from build123d import *

# Parameters (mm, degrees)
F1_W     = 100
F1_H     = 10
F2_DEPTH = 10
F3_R     = 2
F5_COUNT = 4
F6_W     = 15
F6_H     = 15
F6_W_2   = 10
F6_H_2   = 10
F7_DEPTH = 10
F8_DEPTH = 25.4


with BuildPart() as f2:
    # F1 (on Top) → F2 (new body)
    with BuildSketch(Plane.XY):
        Rectangle(F1_W, F1_H)
    extrude(amount=F2_DEPTH)

    # F3
    f3_edges = [f2.edges().sort_by_distance(p)[0] for p in [
        (50, -5, 5),
        (50, 5, 5),
        (50, 0, 0),
        (50, 0, 10),
        (-50, 5, 5),
        (-50, -5, 5),
        (-50, 0, 0),
        (-50, 0, 10),
    ]]
    fillet(f3_edges, radius=F3_R)

    # F5: F2 ×4 about axis
    f5_axis = Axis((0, 0, 17.9461631924), (0, 0, 1))


with BuildPart() as f2_1:
    add(f2.part)
    for i in range(1, F5_COUNT):
        add(f2.part.rotate(f5_axis, i * 360 / F5_COUNT))

    # F6 (on Top) → F7 (join)
    with BuildSketch(Plane.XY):
        Rectangle(F6_W, F6_H)
        Rectangle(F6_W_2, F6_H_2, mode=Mode.SUBTRACT)
    extrude(amount=F7_DEPTH)

    # F6 (on Top) → F8 (cut)
    with BuildSketch(Plane.XY):
        Rectangle(F6_W_2, F6_H_2)
    extrude(amount=F8_DEPTH, mode=Mode.SUBTRACT)


solid = f2_1.part
Verification items for the finished model (mm, model axes). A direction names the side the tool comes from. Coordinates: 2 decimals unless noted, no trailing zeros. Loops run counter-clockwise (first coordinate to the right, second up) from the corner with the lowest first, then second, coordinate; pieces in that order, holes last. Notation, with made-up numbers: (-9.5, -11) -> (36.5, -11) arc R18 ccw to (36.5, 2) -> close; hole circle Ø7 at (35.5, -31). An arc over 180 degrees is marked (long way). Answer as a JSON object with one key per item and string values. Group by question number.
Item 1: Tool access check on faces 4 (the flat face through (-7.5, -6, 5)), 5 (the flat face through (7.5, 6, 5)), 6 (the flat face through (-5, 27, 5)), 7 (the flat face through (0, 5, 5)). Record the directions out of +Z, -Z, +X, -X, +Y, -Y that give a thin tool (end or side, any length) a straight path to the whole face; none if there is none.
Item 2: Depth check by flat-ended pin: pin 1 (2 mm diameter, centred on x = -6.5, z = 6, fed in from -Y); pin 2 (1.5 mm diameter, centred on x = -20.5, z = 2.5, fed in from +Y); pin 3 (1.2 mm diameter, centred on x = 6.5, z = 7, fed in from +Y). Enter the tip coordinate at first touch or a pass-through.
Item 3: Sectioned sample at B-B on y = -23.5. Record the boundary of the cut face in (x, z), plus the area to 3 significant figures.
Item 4: Scan lines: probe 1 along X at (y, z) = (1, 7.5); probe 2 along X at (y, z) = (18, 6.5). Record each from-to range of solid material in increasing order.
Item 5: Mould release check, pull along Y, two halves, no side actions. Record for faces 1 (the flat face through (0, -5, 5)), 2 (the flat face through (-6, -7.5, 5)), 3 (the flat face through (7.5, -6, 5)): +Y half, -Y half, draft (parallel to the pull), parting line (faces both ways), or undercut.
Evaluation:
{
 "1": {"face 4": "+Z, -Z, -X, -Y", "face 5": "+Z, -Z, +X, +Y", "face 6": "+Z, -Z, -X, +Y", "face 7": "+Z, -Z"},
 "2": {"pin 1": "stops at y = -7.5", "pin 2": "stops at y = 5", "pin 3": "stops at y = 7.5"},
 "3": {"outline": "(-5, 0) -> (5, 0) -> (5, 10) -> (-5, 10) -> close", "area": "100 mm²"},
 "4": {"probe 1": "x = -50 to -5, 5 to 50", "probe 2": "x = -5 to 5"},
 "5": {"face 1": "undercut", "face 2": "-Y half", "face 3": "draft"}
}
